from build123d import *

# Parameters (mm, degrees)
BOSS_EXTRUDE1_DEPTH = 19.05


with BuildPart() as part:
    # Sketch1 → Boss-Extrude1 (new body)
    with BuildSketch(Plane.XY):
        with BuildLine():
            Line((-37.913782616, 3.762324776), (-42.067935824, -38.1))
            Line((-42.067935824, -38.1), (-42.067935824, -47.807493339))
            Line((-42.067935824, -47.807493339), (42.067935824, -47.807493339))
            Line((42.067935824, -47.807493339), (42.067935824, -38.1))
            Line((42.067935824, -38.1), (37.913782616, 3.762324776))
            ThreePointArc((37.913782616, 3.762324776), (0, 38.1), (-37.913782616, 3.762324776))
        make_face()
        with BuildLine():
            Line((-37.412264152, -1.987137644), (-40.995876955, -38.1))
            Line((-40.995876955, -38.1), (-40.995876955, -46.6725))
            Line((-40.995876955, -46.6725), (40.995876955, -46.6725))
            Line((40.995876955, -46.6725), (40.995876955, -38.099992109))
            Line((40.995876955, -38.099992109), (37.412264425, -1.987132504))
            ThreePointArc((37.412264425, -1.987132504), (-2.574e-06, 37.465), (-37.412264152, -1.987137644))
        make_face(mode=Mode.SUBTRACT)
    extrude(amount=BOSS_EXTRUDE1_DEPTH)


solid = part.part
Can you work these out from the model? Positions are in its coordinate system, mm. A direction names the side the tool comes from. Give positions to 0.01 mm unless a question says otherwise; leave off trailing zeros. Return JSON: item names as keys, results as strings.
Q1. On a 3-axis mill with a long thin cutter (end or side, diameter ignored), from which of +Z, -Z, +X, -X, +Y, -Y can I reach the whole of each face in a straight line? I mean faces 1 (the face through (-1, -46.672, 9)), 2 (the face through (-38, -1, 0)). Say none if no direction works.
Checks:
{"face 1": "+Z, -Z", "face 2": "-Z, +X, -X, +Y, -Y"}
Q2. I need wall thicknesses on probe 1 along X at (y, z) = (-40, 4.25); probe 2 along X at (y, z) = (-20, 4); probe 3 along Y at (x, z) = (-5.5, 10.5). Which ranges of each line are inside material? Lowest first, please.
Checks:
{"probe 1": "x = -42.07 to -41, 41 to 42.07", "probe 2": "x = -40.27 to -39.2, 39.2 to 40.27", "probe 3": "y = -47.81 to -46.67, 37.06 to 37.7"}
Q3. For pin 1 Ø10 at (x, z) = (-8.5, 9.5) entering from +Y; pin 2 Ø3 at (y, z) = (-14.5, 13) entering from +X; pin 3 Ø1.5 at (x, z) = (7.5, 7.5) entering from +Y, each with a flat end and sliding along its axis, tell me the tip position at first contact or that it passes through.
Checks:
{"pin 1": "stops at y = 37.94", "pin 2": "stops at x = 39.87", "pin 3": "stops at y = 37.5"}
Q4. We'd pull the mould along X, two halves only. Please class faces 3 (the face through (40.996, -42, 9)), 4 (the face through (-39.962, -16.876, 9.392)), 5 (the face through (0.79, 38.09, 9.39)), 6 (the face through (39.23, -20.3, 9.39)): released by +X, released by -X, zero draft, split by the parting line, or undercut.
Checks:
{"face 3": "undercut", "face 4": "released by -X", "face 5": "split by the parting line", "face 6": "undercut"}
